Design review of the part built by this model. Coordinates are the model's own, in mm. A direction names the side the tool comes from. Round coordinates to 2 decimals unless told otherwise and drop trailing zeros. Loops run counter-clockwise (first coordinate to the right, second up) from the corner with the lowest first, then second, coordinate; pieces in that order, holes last. Notation, with made-up numbers: (22, -5) -> (76, -5) arc R13 cw to (76, 8) -> close; hole circle Ø8 at (74, -0.75). An arc over 180 degrees is marked (long way). Use a Markdown table: item, result. Add a question column.
from build123d import *

# Parameters (mm, degrees)
SKETCH_1_W          = 95
SKETCH_1_H          = 120
EXTRUDE_1_DEPTH     = 4
FILLET_1_R          = 3
SKETCH_4_W          = 160
SKETCH_4_H          = 120
SKETCH_4_W_2        = 89
SKETCH_4_H_2        = 114
EXTRUDE_2_DEPTH     = 4
SKETCH_6_R          = 1.25
SKETCH_6_R_2        = 1.250834389
CUT_EXTRUDE_3_DEPTH = 101.480097532
SKETCH_7_W          = 25.2
SKETCH_7_H          = 25
CUT_EXTRUDE_4_DEPTH = 101.480097532
FILLET_3_R          = 3
SKETCH_8_R          = 1.5
CUT_EXTRUDE_5_DEPTH = 101.480097532


with BuildPart() as part:
    # 草图1 → 凸台-拉伸1 (new body)
    with BuildSketch(Plane.XY):
        Rectangle(SKETCH_1_W, SKETCH_1_H)
    extrude(amount=EXTRUDE_1_DEPTH)

    # 圆角1
    fillet_1_edges = [part.edges().sort_by_distance(p)[0] for p in [
        (-47.5, -60, 2),
        (-47.5, 60, 2),
        (47.5, 60, 2),
        (47.5, -60, 2),
    ]]
    fillet(fillet_1_edges, radius=FILLET_1_R)

    # 草图4 → 凸台-拉伸2 (add)
    with BuildSketch(Plane.XY.offset(4)):
        with Locations((-0.5, 0)):
            Rectangle(SKETCH_4_W, SKETCH_4_H)
        Rectangle(SKETCH_4_W_2, SKETCH_4_H_2, mode=Mode.SUBTRACT)
    extrude(amount=-EXTRUDE_2_DEPTH)

    # 草图6 → 切除-拉伸3 (cut, through all)
    with BuildSketch(Plane.XY.offset(4)):
        with Locations((19.425466369, -29.023426318)):
            Circle(SKETCH_6_R)
        with Locations((-8.574533631, -29.023426318)):
            Circle(SKETCH_6_R_2)
        with Locations((-41.074530224, -7.023426499)):
            Circle(SKETCH_6_R)
        with Locations((-41.074530224, -29.023426318)):
            Circle(SKETCH_6_R)
        with Locations((33.925469772, -29.023426318)):
            Circle(SKETCH_6_R)
        with Locations((33.925469772, -7.023426499)):
            Circle(SKETCH_6_R)
    extrude(amount=-CUT_EXTRUDE_3_DEPTH, mode=Mode.SUBTRACT)

    # 草图7 → 切除-拉伸4 (cut, through all)
    with BuildSketch(Plane(origin=(0, 0, 0), x_dir=(-1, 0, 0), z_dir=(0, 0, -1))):
        with Locations((-5.433347592, -28.724095143)):
            Rectangle(SKETCH_7_W, SKETCH_7_H)
    extrude(amount=-CUT_EXTRUDE_4_DEPTH, mode=Mode.SUBTRACT)

    # 圆角3
    fillet_3_edges = [part.edges().sort_by_distance(p)[0] for p in [
        (-7.166652408, -16.224095143, 2),
        (-7.166652408, -41.224095143, 2),
        (18.033347592, -41.224095143, 2),
        (18.033347592, -16.224095143, 2),
        (79.5, -60, 2),
        (-80.5, 60, 2),
        (-80.5, -60, 2),
        (79.5, 60, 2),
    ]]
    fillet(fillet_3_edges, radius=FILLET_3_R)

    # 草图8 → 切除-拉伸5 (cut, through all)
    with BuildSketch(Plane(origin=(0, 0, 0), x_dir=(-1, 0, 0), z_dir=(0, 0, -1))):
        with Locations((70.5, -50)):
            Circle(SKETCH_8_R)
        with Locations((70.5, 50)):
            Circle(SKETCH_8_R)
        with Locations((-69.5, 50)):
            Circle(SKETCH_8_R)
        with Locations((-69.5, -50)):
            Circle(SKETCH_8_R)
    extrude(amount=-CUT_EXTRUDE_5_DEPTH, mode=Mode.SUBTRACT)


solid = part.part
1. Insertion check: P1, Ø1.8, axis at x = 69.5, y = 50, coming from the +Z side. The pin has a flat end and moves straight along its axis. Give the tip position at first contact, or say it passes through.
2. To check wall thickness, follow probe 1 along Y at (x, z) = (69.5, 0.8); probe 2 along Y at (x, z) = (-8.5, 3.35); probe 3 along X at (y, z) = (-6, 2.9). State the ranges of each line that lie inside material, in increasing order. Write a range as from..to.
3. Consider section A-A on x = 8. State the section outline as (y, z) points.
4. Consider section B-B on z = 3.35. Give the number of separate pieces and of enclosed holes in the cut face, plus the area to 3 significant figures.
5. Mouldability with a two-part tool opening along Y and no side actions: class faces 3 (the face through (-2, 1, 0)), 4 (the face through (-2, -60, 2)), 5 (the face through (-2, 60, 2)), 6 (the face through (6, -41.224, 2)) as +Y half, -Y half, draft (parallel to the pull), parting line (faces both ways), or undercut.
6. For faces 1 (the face through (79.5, -1, 2)), 2 (the face through (18.033, -28.86, 1.97)), list the 3-axis set-ups (+Z, -Z, +X, -X, +Y, -Y) from which the entire face can be reached by the end or side of a thin tool; tool diameter is ignored.
Verdict:
| question | item | result |
|---|---|---|
| 1 | P1 | passes through |
| 2 | probe 1 | y = -60..-51.5, -48.5..48.5, 51.5..60 |
| 2 | probe 2 | y = -60..-30.27, -27.77..60 |
| 2 | probe 3 | x = -80.5..-41.79, -40.36..33.21, 34.64..79.5 |
| 3 | outline | (-60, 0) -> (-41.22, 0) -> (-41.22, 4) -> (-60, 4) -> close; (-16.22, 0) -> (60, 0) -> (60, 4) -> (-16.22, 4) -> close |
| 4 | separate pieces | 1 |
| 4 | enclosed holes | 11 |
| 4 | area | 18,500 mm² |
| 5 | face 3 | draft |
| 5 | face 4 | -Y half |
| 5 | face 5 | +Y half |
| 5 | face 6 | undercut |
| 6 | face 1 | +Z, -Z, +X, +Y, -Y |
| 6 | face 2 | +Z, -Z |
